Work out the finished part from the listing and answer in its coordinate system (mm). Face numbers are marked on the shaded views. A direction names the side the tool comes from. Coordinates: 2 decimals unless noted, no trailing zeros. Order: outer loops, then holes, each group sorted by start corner. A loop starts at its lowest first (then second) coordinate and runs counter-clockwise, first axis right, second up. Notation, with made-up numbers: M 21.5,5 L 68.5,5 A29 ccw 68.5,42 Z; hole C 46.25,50 d2. An arc over 180 degrees is marked long. Use a Markdown table: item, result.
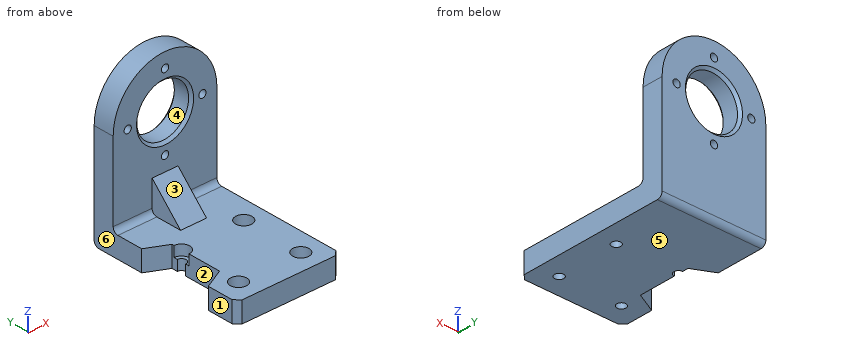
from build123d import *

# Parameters (mm, degrees)
F0_W      = 200
F0_H      = 40
F0_R      = 7
F0_R_2    = 50
F1_DEPTH  = 40
F2_DEPTH  = 300
F3_SIZE   = 5
F4_R      = 8.75
F5_DEPTH  = 40.001
F4_R_2    = 15.75
F6_DEPTH  = 20
F7_SIZE   = 10
F8_R      = 10
F10_DEPTH = 25
F13_DEPTH = 40.001
F14_R     = 10


with BuildPart() as f1:
    # F0 (on Front) → F1 (new body)
    with BuildSketch(Plane.XZ):
        with Locations((0, 20)):
            Rectangle(F0_W, F0_H)
        with BuildLine():
            Line((-100, 200), (-100, 40))
            Line((-100, 40), (100, 40))
            Line((100, 40), (100, 200))
            ThreePointArc((100, 200), (0, 300), (-100, 200))
        make_face()
        with Locations((0, 128)):
            Circle(F0_R, mode=Mode.SUBTRACT)
        with Locations((-72, 200)):
            Circle(F0_R, mode=Mode.SUBTRACT)
        with Locations((0, 200)):
            Circle(F0_R_2, mode=Mode.SUBTRACT)
        with Locations((72, 200)):
            Circle(F0_R, mode=Mode.SUBTRACT)
        with Locations((0, 272)):
            Circle(F0_R, mode=Mode.SUBTRACT)
    extrude(amount=F1_DEPTH)

    # F0 (on Front) → F2 (join)
    with BuildSketch(Plane.XZ):
        with Locations((0, 20)):
            Rectangle(F0_W, F0_H)
    extrude(amount=F2_DEPTH)

    # F3
    f3_edges = [f1.edges().sort_by_distance(p)[0] for p in [
        (-50, -40, 200),
        (-50, 0, 200),
    ]]
    chamfer(f3_edges, length=F3_SIZE)

    # F4 (on face) → F5 (cut, through all)
    with BuildSketch(Plane.XY.offset(40)):
        with Locations((60, -140)):
            Circle(F4_R)
        with Locations((-60, -140)):
            Circle(F4_R)
        with Locations((60, -260)):
            Circle(F4_R)
        with Locations((-60, -260)):
            Circle(F4_R)
    extrude(amount=-F5_DEPTH, mode=Mode.SUBTRACT)

    # F4 (on face) → F6 (cut)
    with BuildSketch(Plane.XY.offset(40)):
        with Locations((-60, -140)):
            Circle(F4_R_2)
        with Locations((-60, -140)):
            Circle(F4_R, mode=Mode.SUBTRACT)
        with Locations((60, -140)):
            Circle(F4_R_2)
        with Locations((60, -140)):
            Circle(F4_R, mode=Mode.SUBTRACT)
        with Locations((60, -260)):
            Circle(F4_R_2)
        with Locations((60, -260)):
            Circle(F4_R, mode=Mode.SUBTRACT)
        with Locations((-60, -260)):
            Circle(F4_R_2)
        with Locations((-60, -260)):
            Circle(F4_R, mode=Mode.SUBTRACT)
    extrude(amount=-F6_DEPTH, mode=Mode.SUBTRACT)

    # F7
    f7_edges = [f1.edges().sort_by_distance(p)[0] for p in [
        (-100, -300, 20),
        (100, -300, 20),
    ]]
    chamfer(f7_edges, length=F7_SIZE)

    # F8
    f8_edges = [f1.edges().sort_by_distance(p)[0] for p in [
        (0, 0, 0),
    ]]
    fillet(f8_edges, radius=F8_R)

    # F9 (on Right) → F10 (join, symmetric)
    with BuildSketch(Plane.YZ):
        Polygon((-40, 100), (-100, 40), (-40, 40), align=None)
    extrude(amount=F10_DEPTH, both=True)

    # F12 (on offset) → F13 (cut, through all)
    with BuildSketch(Plane.XY.offset(40)):
        Polygon((-100, -100), (-100, -240), (-60, -220), (-60, -120), align=None)
    extrude(amount=-F13_DEPTH, mode=Mode.SUBTRACT)

    # F14
    f14_edges = [f1.edges().sort_by_distance(p)[0] for p in [
        (62.5, -40, 40),
        (-62.5, -40, 40),
    ]]
    fillet(f14_edges, radius=F14_R)


solid = f1.part
1. For a pull along Z with two mould halves and no side action, classify the marked faces 3, 4, 5 and 6 as +Z half, -Z half, draft (parallel to the pull), parting line (faces both ways), or undercut.
Answers below:
| item | result |
|---|---|
| face 3 | +Z half |
| face 4 | undercut |
| face 5 | -Z half |
| face 6 | draft |
2. Flat-ended cylindrical pins translate along their axes: P1, Ø8, axis at x = 46.5, y = -167.5, coming from the -Z side; P2, Ø8, axis at x = 61, z = 64, coming from the -Y side; P3, Ø25, axis at x = 59, y = -264.5, coming from the +Z side; P4, Ø18, axis at y = -83.5, z = 64, coming from the -X side. Find the tip coordinate at first contact, or state that the pin passes through.
Answers below:
| item | result |
|---|---|
| P1 | z = 0 |
| P2 | y = -40 |
| P3 | z = 40 |
| P4 | x = -25 |
3. Section D-D on z = 28 is taken. Determine the outline of the cut face in (x, y), then the cut area to 3 significant figures.
Answers below:
| item | result |
|---|---|
| outline | M -100,-290 L -90,-300 L 90,-300 L 100,-290 L 100,0 L -100,0 L -100,-100 L -60,-120 L -60,-124.25 A15.75 cw -60,-155.75 L -60,-220 L -100,-240 Z; hole C -60,-260 d31.5; hole C 60,-260 d31.5; hole C 60,-140 d31.5 |
| area | 52,400 mm² |
4. Section A-A on x = 0 is taken. Determine the outline of the cut face in (y, z), then the cut area to 3 significant figures.
Answers below:
| item | result |
|---|---|
| outline | M -300,0 L -10,0 A10 ccw 0,10 L 0,121 L -40,121 L -40,100 L -100,40 L -300,40 Z; M -40,135 L 0,135 L 0,145 L -5,150 L -35,150 L -40,145 Z; M -40,255 L -35,250 L -5,250 L 0,255 L 0,265 L -40,265 Z; M -40,279 L 0,279 L 0,300 L -40,300 Z |
| area | 19,000 mm² |
5. Section C-C on x = 60 is taken. Determine the outline of the cut face in (y, z).
Answers below:
| item | result |
|---|---|
| outline | M -300,0 L -268.75,0 L -268.75,20 L -275.75,20 L -275.75,40 L -300,40 Z; M -251.25,0 L -148.75,0 L -148.75,20 L -155.75,20 L -155.75,40 L -244.25,40 L -244.25,20 L -251.25,20 Z; M -131.25,0 L -10,0 A10 ccw 0,10 L 0,280 L -40,280 L -40,50 A10 cw -50,40 L -124.25,40 L -124.25,20 L -131.25,20 Z |
6. For the marked faces 1 and 2, determine the directions among +Z, -Z, +X, -X, +Y, -Y from which every point of the face is accessible in a straight line to the end or side of a thin tool.
Answers below:
| item | result |
|---|---|
| face 1 | +Z, -Z, -X, +Y, -Y |
| face 2 | +Z, -Z, -X |
7. Find the intervals of material crossed by probe 1 along Y at (x, z) = (60, 15); probe 2 along Z at (x, y) = (0, -19.5); probe 3 along Y at (x, z) = (60, 6.75), in increasing order.
Answers below:
| item | result |
|---|---|
| probe 1 | -300 to -268.75, -251.25 to -148.75, -131.25 to 0 |
| probe 2 | 0 to 121, 135 to 150, 250 to 265, 279 to 300 |
| probe 3 | -300 to -268.75, -251.25 to -148.75, -131.25 to -0.54 |
8. Section B-B on y = -260 is taken. Determine the outline of the cut face in (x, z), then the cut area to 3 significant figures.
Answers below:
| item | result |
|---|---|
| outline | M -100,0 L -68.75,0 L -68.75,20 L -75.75,20 L -75.75,40 L -100,40 Z; M -51.25,0 L 51.25,0 L 51.25,20 L 44.25,20 L 44.25,40 L -44.25,40 L -44.25,20 L -51.25,20 Z; M 68.75,0 L 100,0 L 100,40 L 75.75,40 L 75.75,20 L 68.75,20 Z |
| area | 6,040 mm² |
